Input: part model. Units: mm. Frame: model coordinates. Face numbers are marked on the shaded views. A direction names the side the tool comes from. Give positions to 0.01 mm unless a question says otherwise; leave off trailing zeros. Loops run counter-clockwise (first coordinate to the right, second up) from the corner with the lowest first, then second, coordinate; pieces in that order, holes last. Notation, with made-up numbers: M 62.25,1 L 88.25,1 A11 cw 88.25,5 Z; hole C 80.25,22 d6. An arc over 180 degrees is marked long. Return JSON: item names as keys, results as strings. Group by question number.
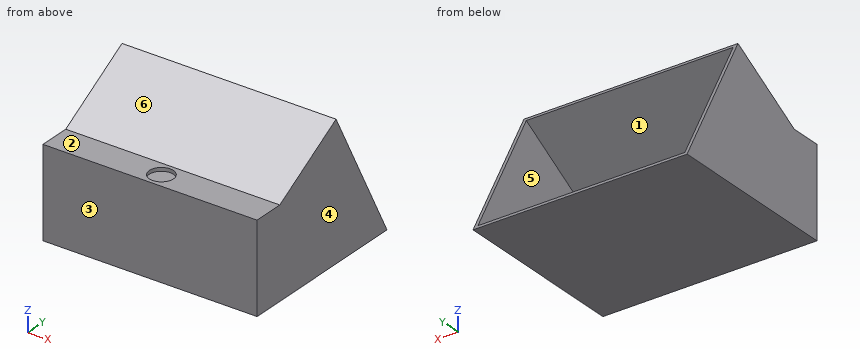
```python
from build123d import *

# Parameters (mm, degrees)
F1_DEPTH = 480
F2_T     = -8
F3_R     = 27
F4_DEPTH = 25


with BuildPart() as f1:
    # F0 (on Right) → F1 (new body)
    with BuildSketch(Plane.YZ):
        Polygon((0, 200), (0, 0), (400, 0), (243.2050807569, 300), (70, 200), align=None)
    extrude(amount=F1_DEPTH)

    # F2
    f2_openings = [f1.faces().sort_by_distance(p)[0] for p in [
        (240, 321.60254, 150),
    ]]
    offset(amount=F2_T, openings=f2_openings, kind=Kind.INTERSECTION)

    # F3 (on face) → F4 (cut)
    with BuildSketch(Plane.XY.offset(200)):
        with Locations((240, 35)):
            Circle(F3_R)
    extrude(amount=-F4_DEPTH, mode=Mode.SUBTRACT)


solid = f1.part
```
Item 1: First-contact query: pin 1 Ø12 at (x, y) = (337, 308.5) entering from +Z; pin 2 Ø12 at (x, z) = (368.5, 148) entering from +Y; pin 3 Ø5 at (x, z) = (323.5, 238) entering from +Y. Flat tips, straight axial feed; report the tip coordinate or a pass-through.
Item 2: Pull-direction query (Z, two-part tool) for the marked faces 4, 5 and 6; classes: pulls with the +Z half, pulls with the -Z half, needs draft (parallel to the pull), parting line crosses it, or undercut.
Item 3: Section C-C, the plane z = 162.5. Return loops of the section in (x, y).
Item 4: Section B-B, the plane y = 35. Return loops of the section in (x, z), then the cut area to 3 significant figures.
Item 5: Section A-A, the plane x = 442.5. Return loops of the section in (y, z).
Item 6: Material intervals for line 1 (X direction, y = 175, z = 81.5); line 2 (X direction, y = 35, z = 194.75); line 3 (Z direction, x = 32, y = 53.5), sorted ascending. Write a range as from..to.
Item 7: Section D-D, the plane x = 220.5. Return loops of the section in (y, z).
Item 8: Reachability of the marked faces 1, 2 and 3 from +Z, -Z, +X, -X, +Y, -Y: full face, straight path, thin tool, end or side. Return the list, or none.
Answer below:
{
 "1": {"pin 1": "z = 8", "pin 2": "y = 8", "pin 3": "y = 156.15"},
 "2": {"face 4": "needs draft", "face 5": "undercut", "face 6": "pulls with the +Z half"},
 "3": {"outline": "M 0,0 L 480,0 L 480,315.07 L 472,315.07 L 472,8 L 8,8 L 8,315.07 L 0,315.07 Z"},
 "4": {"outline": "M 0,0 L 480,0 L 480,200 L 267,200 L 267,192 L 472,192 L 472,8 L 8,8 L 8,192 L 213,192 L 213,200 L 0,200 Z", "area": "10,200 mm^2"},
 "5": {"outline": "M 0,0 L 400,0 L 395.82,8 L 8,8 L 8,192 L 72.14,192 L 246.91,292.9 L 243.21,300 L 70,200 L 0,200 Z"},
 "6": {"line 1": "0..8, 472..480", "line 2": "0..213, 267..480", "line 3": "0..8, 192..200"},
 "7": {"outline": "M 0,0 L 400,0 L 395.82,8 L 8,8 L 8,192 L 16.33,192 L 16.33,200 L 0,200 Z; M 53.67,192 L 72.14,192 L 246.91,292.9 L 243.21,300 L 70,200 L 53.67,200 Z"},
 "8": {"face 1": "+Y", "face 2": "+Z, +X, -X, -Y", "face 3": "+Z, -Z, +X, -X, -Y"}
}
